Model file for the job. Use its own axes, mm. A direction names the side the tool comes from. Round coordinates to 2 decimals unless told otherwise and drop trailing zeros. Order: outer loops, then holes, each group sorted by start corner. A loop starts at its lowest first (then second) coordinate and runs counter-clockwise, first axis right, second up. Notation, with made-up numbers: (-37.5, -37) -> (-6.5, -37) arc R19 ccw to (-6.5, -15) -> close; hole circle Ø9 at (23, 37). An arc over 180 degrees is marked (long way). Put each result on its own line as item: value. Start each with the question number.
Q1. Cut at D-D, the plane x = 0. List the corners of the cut face in (y, z).
Q2. Flat gauge pins, fed straight in: P1, Ø1.6, axis at x = -78.5, y = 2, coming from the -Z side; P2, Ø3.5, axis at x = -80, z = 0, coming from the -Y side. Where does each tip first touch, or does it go through?
Q3. Pull direction X, two halves, no side cores. Call faces 1 (the face through (-62, 0, -43)), 2 (the face through (-61.75, 1.61, -127.22)), 3 (the face through (-82, 2, 0)): released by +X, released by -X, zero draft, split by the parting line, or undercut.
Q4. Probe L1, parallel to X at y = 0.95, z = -37.5; L2, parallel to Z at x = -15.5, y = 2.35; L3, parallel to X at y = 2.65, z = -68. List the from-to ranges inside material, lowest first.
Q5. 3-axis set-ups, long thin cutter, end or side, ignore diameter. For faces 4 (the face through (-2.9, 1.61, -8.86)), 5 (the face through (-102.924, 1.612, 6.859)): which of +Z, -Z, +X, -X, +Y, -Y reach the whole face in a straight line?
Q6. Cut at B-B, the plane x = -48. List the corners of the cut face in (y, z).
Q7. Cut at C-C, the plane z = 0. State how many separate pieces and enclosed holes the cut face has, and give its area (3 significant figures).
Q8. Cut at A-A, the plane z = -61. List the corners of the cut face in (x, y), and give its area (3 significant figures).
from build123d import *

# Parameters (mm, degrees)
SKETCH1_R           = 2
BOSS_EXTRUDE1_DEPTH = 3.18
FILLET2_R           = 4
FILLET4_R           = 3
FILLET5_R           = 2


with BuildPart() as part:
    # Sketch1 → Boss-Extrude1 (new body)
    with BuildSketch(Plane(origin=(0, 0, 0), x_dir=(1, 0, 0), z_dir=(0, 1, 0))):
        Polygon((-16, -8), (6, -8), (6, 33.34843691), (-61.475760907, 128.370940703), (-81.524239093, 119.312324779), (-104.126855641, 18.58956294), (-104.126855641, -8), (-86.093666761, -8), align=None)
        with Locations(Location((-16, 0, 0), (0, 0, 90))):
            Circle(SKETCH1_R, mode=Mode.SUBTRACT)
        with Locations(Location((0, 0, 0), (0, 0, 90))):
            Circle(SKETCH1_R, mode=Mode.SUBTRACT)
        with Locations(Location((-67.5, 116.913429511, 0), (0, 0, 90))):
            Circle(SKETCH1_R, mode=Mode.SUBTRACT)
        with Locations(Location((-32, 0, 0), (0, 0, 90))):
            Circle(SKETCH1_R, mode=Mode.SUBTRACT)
        with Locations(Location((-48, 0, 0), (0, 0, 90))):
            Circle(SKETCH1_R, mode=Mode.SUBTRACT)
        with Locations(Location((-64, 0, 0), (0, 0, 90))):
            Circle(SKETCH1_R, mode=Mode.SUBTRACT)
        with Locations(Location((-80, 0, 0), (0, 0, 90))):
            Circle(SKETCH1_R, mode=Mode.SUBTRACT)
        with Locations(Location((-96, 0, 0), (0, 0, 90))):
            Circle(SKETCH1_R, mode=Mode.SUBTRACT)
        with Locations(Location((-97.021679837, 31.983686003, 0), (0, 0, 90))):
            Circle(SKETCH1_R, mode=Mode.SUBTRACT)
        Polygon((-63.513465031, 117.423073167), (-2, 30.796951643), (-2, 8), (-60.237701437, 8), align=None, mode=Mode.SUBTRACT)
        Polygon((-68.241285453, 8), (-98.304243511, 8), (-74.592422981, 113.66564481), (-71.44710907, 115.086809569), align=None, mode=Mode.SUBTRACT)
    extrude(amount=BOSS_EXTRUDE1_DEPTH)

    # Fillet2
    fillet2_edges = [part.edges().sort_by_distance(p)[0] for p in [
        (6, 1.59, 8),
        (-104.126855641, 1.59, 8),
        (-104.126855641, 1.59, -18.58956294),
        (-81.524239093, 1.59, -119.312324779),
        (-61.475760907, 1.59, -128.370940703),
        (6, 1.59, -33.34843691),
    ]]
    fillet(fillet2_edges, radius=FILLET2_R)

    # Fillet4
    fillet4_edges = [part.edges().sort_by_distance(p)[0] for p in [
        (-98.304243511, 1.59, -8),
        (-68.241285453, 1.59, -8),
        (-63.513465031, 1.59, -117.423073167),
        (-60.237701437, 1.59, -8),
        (-2, 1.59, -8),
        (-2, 1.59, -30.796951643),
    ]]
    fillet(fillet4_edges, radius=FILLET4_R)

    # Fillet5
    # the kernel refuses this fillet: 2 mm, written as the material it adds along each edge
    with BuildSketch(Plane(origin=(-71.44710907, 0, -115.086809569), x_dir=(0.02992327493551802, 0, 0.9995521985454954), z_dir=(0, 1, 0))) as fillet5_piece_1:
        with BuildLine():
            CenterArc((FILLET5_R * 1.49944843897, -FILLET5_R), FILLET5_R, 90, 112.600412538)
            Line((FILLET5_R * 0.576240988861, -FILLET5_R * 1.3843019699), (0, 0))
            Line((0, 0), (FILLET5_R * 1.49944843897, 0))
        make_face()
    extrude(amount=3.18)
    with BuildSketch(Plane(origin=(-74.592422981, 0, -113.66564481), x_dir=(-0.21895888286608584, 0, 0.9757340865287201), z_dir=(0, 1, 0))) as fillet5_piece_2:
        with BuildLine():
            CenterArc((FILLET5_R * 0.498984426224, FILLET5_R), FILLET5_R, 216.963036407, 53.036963593)
            Line((-FILLET5_R * 0.300039170379, FILLET5_R * 0.39870033089), (0, 0))
            Line((0, 0), (FILLET5_R * 0.498984426224, 0))
        make_face()
    extrude(amount=3.18)


solid = part.part
Ans:
1. outline: (0, -41.8) -> (3.18, -41.8) -> (3.18, -2) -> (0, -2) -> close; (0, 2) -> (3.18, 2) -> (3.18, 8) -> (0, 8) -> close
2. P1: stops at z = -121.04
2. P2: passes through
3. face 1: zero draft
3. face 2: split by the parting line
3. face 3: undercut
4. L1: x = -99.88 to -91.68, -69.12 to -61.12, -6.76 to 3.05
4. L2: z = -63.63 to -49.81, -8 to -1.94, 1.94 to 8
4. L3: x = -93.04 to -84.84, -70.04 to -62.03, -28.42 to -18.61
5. face 4: +Y, -Y
5. face 5: +Z, -X, +Y, -Y
6. outline: (0, -109.39) -> (3.18, -109.39) -> (3.18, -95.58) -> (0, -95.58) -> close; (0, -8) -> (3.18, -8) -> (3.18, -2) -> (0, -2) -> close; (0, 2) -> (3.18, 2) -> (3.18, 8) -> (0, 8) -> close
7. separate pieces: 8
7. enclosed holes: 0
7. area: 261 mm^2
8. outline: (-94.61, 0) -> (-86.41, 0) -> (-86.41, 3.18) -> (-94.61, 3.18) -> close; (-69.83, 0) -> (-61.82, 0) -> (-61.82, 3.18) -> (-69.83, 3.18) -> close; (-23.45, 0) -> (-13.64, 0) -> (-13.64, 3.18) -> (-23.45, 3.18) -> close
8. area: 82.7 mm^2
